```python
from build123d import *

# Parameters (mm, degrees)
SKETCH1_W           = 128
SKETCH1_H           = 65.5
BOSS_EXTRUDE1_DEPTH = 1.5
SKETCH2_R           = 1.6
CUT_EXTRUDE2_DEPTH  = 72.908361823
SKETCH3_W           = 105
SKETCH3_H           = 18
BOSS_EXTRUDE2_DEPTH = 1
SKETCH4_R           = 8.1
BOSS_EXTRUDE4_DEPTH = 24.5


with BuildPart() as part:
    # Sketch1 → Boss-Extrude1 (new body)
    with BuildSketch(Plane(origin=(0, 0, 0), x_dir=(1, 0, 0), z_dir=(0, 1, 0))):
        Rectangle(SKETCH1_W, SKETCH1_H)
    extrude(amount=BOSS_EXTRUDE1_DEPTH)

    # Sketch2 → Cut-Extrude2 (cut, through all)
    with BuildSketch(Plane(origin=(0, 0, 0), x_dir=(1, 0, 0), z_dir=(0, 1, 0))):
        with Locations(Location((-51.4, -28.75, 0), (0, 0, 270))):
            Circle(SKETCH2_R)
        with Locations(Location((0, -28.75, 0), (0, 0, 270))):
            Circle(SKETCH2_R)
        with Locations(Location((51.4, -28.75, 0), (0, 0, 270))):
            Circle(SKETCH2_R)
        with Locations(Location((-51.4, 8.55, 0), (0, 0, 270))):
            Circle(SKETCH2_R)
        with Locations(Location((0, 8.55, 0), (0, 0, 270))):
            Circle(SKETCH2_R)
        with Locations(Location((51.4, 8.55, 0), (0, 0, 270))):
            Circle(SKETCH2_R)
    extrude(amount=CUT_EXTRUDE2_DEPTH, mode=Mode.SUBTRACT)

    # Sketch3 → Boss-Extrude2 (add)
    with BuildSketch(Plane.XZ):
        with Locations((0, 10.75)):
            Rectangle(SKETCH3_W, SKETCH3_H)
    extrude(amount=BOSS_EXTRUDE2_DEPTH)

    # Sketch4 → Boss-Extrude4 (add)
    with BuildSketch(Plane(origin=(0, 0, -32.75), x_dir=(-1, 0, 0), z_dir=(0, 0, -1))):
        with Locations(Location((-48, 0.5, 0), (0, 0, 183.539026459))):
            Circle(SKETCH4_R)
        with Locations(Location((-31.7, 0.5, 0), (0, 0, 183.539026459))):
            Circle(SKETCH4_R)
        with Locations(Location((-15.4, 0.5, 0), (0, 0, 183.539026459))):
            Circle(SKETCH4_R)
        with Locations(Location((15.4, 0.5, 0), (0, 0, 183.539026459))):
            Circle(SKETCH4_R)
        with Locations(Location((31.7, 0.5, 0), (0, 0, 183.539026459))):
            Circle(SKETCH4_R)
        with Locations(Location((48, 0.5, 0), (0, 0, 183.539026459))):
            Circle(SKETCH4_R)
    extrude(amount=BOSS_EXTRUDE4_DEPTH)


solid = part.part
```
Read the model definition and answer for the solid it produces. Units are mm, in the model's axes. A direction names the side the tool comes from. Round coordinates to 2 decimals unless told otherwise and drop trailing zeros. Write each loop counter-clockwise with the first axis right and the second up, starting at its lowest first coordinate (ties: lowest second). Pieces come first, ordered by that corner, then holes. Notation, with made-up numbers: (-2.75, 29.25) -> (2.25, 29.25) arc R28 ccw to (2.25, 50.25) -> close; hole circle Ø1 at (46, 76). An arc over 180 degrees is marked (long way). Answer in a Markdown table with one row per item. Add a question column.
1) Given P1, Ø2.5, axis at x = -35.5, y = -3, coming from the +Z side; P2, Ø4, axis at x = 30, z = -6, coming from the +Y side; P3, Ø6, axis at x = 24, z = -36.5, coming from the -Y side, each flat-ended and moving along its own axis, determine where each tip first touches the part or whether it passes through.
2) Determine the mould class of faces 1 (the face through (15, 0, -57.25)), 2 (the face through (0.481, 0.74, -7.024)), 3 (the face through (55.56, -2.41, -44.83)) for opening direction Z: pulls with the +Z half, pulls with the -Z half, needs draft (parallel to the pull), parting line crosses it, or undercut.
3) Find section A-A, the plane z = 28.75. Determine the outline of the cut face in (x, y), and give its area (3 significant figures).
4) Which of the six approach directions +Z, -Z, +X, -X, +Y, -Y give full straight-line access (tool end or side, diameter ignored) to faces 4 (the face through (-48, -4, -32.75)), 5 (the face through (15, 5, -32.75)), 6 (the face through (0.07, 0.74, 27.15))?
5) Find section D-D, the plane z = 10. Determine the outline of the cut face in (x, y).
6) Find section B-B, the plane y = 6.75. Determine the outline of the cut face in (x, z), and give its area (3 significant figures).
7) Find section C-C, the plane x = -48. Determine the outline of the cut face in (y, z), and give its area (3 significant figures).
8) Consider line 1 (Z direction, x = 51.4, y = 1.1); line 2 (X direction, y = 0.4, z = -8.55); line 3 (Z direction, x = 0, y = 0.85). Determine where each line is inside the solid, lowest interval first.
Findings below:
| question | item | result |
|---|---|---|
| 1 | P1 | z = -32.75 |
| 1 | P2 | y = 1.5 |
| 1 | P3 | y = -6.1 |
| 2 | face 1 | pulls with the -Z half |
| 2 | face 2 | undercut |
| 2 | face 3 | needs draft |
| 3 | outline | (-64, 0) -> (-53, 0) -> (-53, 1.5) -> (-64, 1.5) -> close; (-49.8, 0) -> (-1.6, 0) -> (-1.6, 1.5) -> (-49.8, 1.5) -> close; (1.6, 0) -> (49.8, 0) -> (49.8, 1.5) -> (1.6, 1.5) -> close; (53, 0) -> (64, 0) -> (64, 1.5) -> (53, 1.5) -> close |
| 3 | area | 178 mm² |
| 4 | face 4 | +X, -X, -Y |
| 4 | face 5 | +Z, +X, -X, +Y |
| 4 | face 6 | +Y, -Y |
| 5 | outline | (-64, 0) -> (-52.5, 0) -> (-52.5, -1) -> (52.5, -1) -> (52.5, 0) -> (64, 0) -> (64, 1.5) -> (-64, 1.5) -> close |
| 6 | outline | (-53.15, -57.25) -> (-42.85, -57.25) -> (-42.85, -32.75) -> (-53.15, -32.75) -> close; (-36.85, -57.25) -> (-26.55, -57.25) -> (-26.55, -32.75) -> (-36.85, -32.75) -> close; (-20.55, -57.25) -> (-10.25, -57.25) -> (-10.25, -32.75) -> (-20.55, -32.75) -> close; (10.25, -57.25) -> (20.55, -57.25) -> (20.55, -32.75) -> (10.25, -32.75) -> close; (26.55, -57.25) -> (36.85, -57.25) -> (36.85, -32.75) -> (26.55, -32.75) -> close; (42.85, -57.25) -> (53.15, -57.25) -> (53.15, -32.75) -> (42.85, -32.75) -> close |
| 6 | area | 1,510 mm² |
| 7 | outline | (-7.6, -57.25) -> (8.6, -57.25) -> (8.6, -32.75) -> (1.5, -32.75) -> (1.5, 32.75) -> (0, 32.75) -> (0, 19.75) -> (-1, 19.75) -> (-1, 1.75) -> (0, 1.75) -> (0, -32.75) -> (-7.6, -32.75) -> close |
| 7 | area | 513 mm² |
| 8 | line 1 | -57.25 to -10.15, -6.95 to 27.15, 30.35 to 32.75 |
| 8 | line 2 | -64 to -53, -49.8 to -1.6, 1.6 to 49.8, 53 to 64 |
| 8 | line 3 | -32.75 to -10.15, -6.95 to 27.15, 30.35 to 32.75 |
